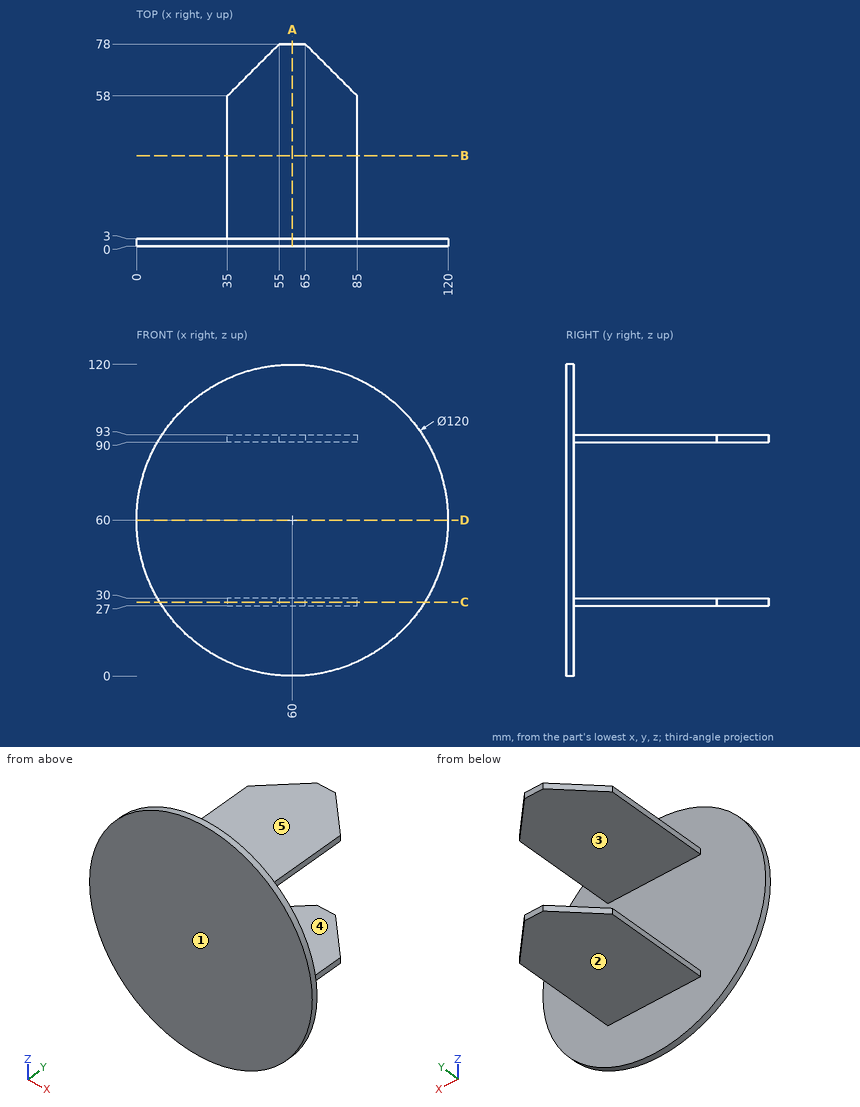
Study the drawing (mm; zero at the part's minimum x, y, z) and answer. A direction names the side the tool comes from. Coordinates: 2 decimals unless noted, no trailing zeros. Write each loop counter-clockwise with the first axis right and the second up, starting at its lowest first coordinate (ties: lowest second). Pieces come first, ordered by that corner, then holes. Notation, with made-up numbers: (21.25, 47.25) - (49.25, 47.25) arc R29 ccw to (49.25, 77.25) - close; hole circle Ø4 at (35, -7). An arc over 180 degrees is marked (long way). Return JSON: item names as keys, results as strings. Group by question number.
1. A cutting plane is placed at C-C, the plane z = 28.5. Determine the outline of the cut face in (x, y), plus the area to 3 significant figures.
2. Which of the six approach directions +Z, -Z, +X, -X, +Y, -Y give full straight-line access (tool end or side, diameter ignored) to the marked faces 4 and 5?
3. A cutting plane is placed at B-B, the plane y = 35. Determine the outline of the cut face in (x, z), plus the area to 3 significant figures.
4. Given pin 1 (2.5 mm diameter, centred on y = 22.5, z = 28, fed in from -X); pin 2 (15 mm diameter, centred on x = 49, y = 40.5, fed in from +Z); pin 3 (6 mm diameter, centred on x = 19.5, z = 57, fed in from +Y), each flat-ended and moving along its own axis, determine where each tip first touches the part or whether it passes through.
5. A cutting plane is placed at D-D, the plane z = 60. Determine the outline of the cut face in (x, y), plus the area to 3 significant figures.
6. Determine the mould class of the marked faces 1, 2 and 3 for opening direction Z: released by +Z, released by -Z, zero draft, split by the parting line, or undercut.
7. Straight lines are drawn through the part: L1, parallel to Z at x = 45, y = 36; L2, parallel to X at y = 56, z = 90.5; L3, parallel to Y at x = 33.5, z = 94. For each, find the intervals that lie inside material, in ascending order.
8. A cutting plane is placed at A-A, the plane x = 60. Determine the outline of the cut face in (y, z).
Ans:
{
 "1": {"outline": "(8.93, 0) - (111.07, 0) - (111.07, 3) - (85, 3) - (85, 58) - (65, 78) - (55, 78) - (35, 58) - (35, 3) - (8.93, 3) - close", "area": "3,660 mm²"},
 "2": {"face 4": "+X, -X, +Y", "face 5": "+Z, +X, -X, +Y"},
 "3": {"outline": "(35, 27) - (85, 27) - (85, 30) - (35, 30) - close; (35, 90) - (85, 90) - (85, 93) - (35, 93) - close", "area": "300 mm²"},
 "4": {"pin 1": "x = 35", "pin 2": "z = 93", "pin 3": "y = 3"},
 "5": {"outline": "(0, 0) - (120, 0) - (120, 3) - (0, 3) - close", "area": "360 mm²"},
 "6": {"face 1": "zero draft", "face 2": "released by -Z", "face 3": "undercut"},
 "7": {"L1": "27 to 30, 90 to 93", "L2": "35 to 85", "L3": "0 to 3"},
 "8": {"outline": "(0, 0) - (3, 0) - (3, 27) - (78, 27) - (78, 30) - (3, 30) - (3, 90) - (78, 90) - (78, 93) - (3, 93) - (3, 120) - (0, 120) - close"}
}
